Autodesk Inventor part; units mm, degrees
ref_plane "YZ Plane" through (0, 0, 0) normal (1, 0, 0) x (0, 1, 0)
ref_plane "XZ Plane" through (0, 0, 0) normal (0, 1, 0) x (-1, 0, 0)
ref_plane "XY Plane" through (0, 0, 0) normal (0, 0, 1) x (1, 0, 0)
sketch "Эскиз1" plane through (0, 0, 0) normal (0, 0, 1) x (1, 0, 0)
  line L0 (40, 0) -> (0, 0)
  line L1 (40, 0) -> (40, -6)
  line L2 (0, -6) -> (40, -6)
  line L3 (0, 0) -> (0, -6)
  line L4 (0, 0) -> (0, 20)
  line L5 (0, 20) -> (18.33, 29.326)
  line L6 (40, 0) -> (40, 29.326)
  line L7 (40, 29.326) -> (18.33, 29.326)
  dimension "d0" = 20
extrude "Выдавливание1" add sketch "Эскиз1" along normal blind 6
sketch "Эскиз2" plane through (0, 0, 6) normal (0, 0, 1) x (1, 0, 0)
  line L0 (0, 20) -> (0, -6)
  line L1 (40, 29.326) -> (18.33, 29.326)
  line L2 (18.33, 29.326) -> (0, 20)
  line L3 (18.33, 29.326) -> (0, 20)
  line L4 (0, 8.2778) -> (18.33, 29.326)
  point P0 (0, 0)
extrude "Выдавливание2" cut sketch "Эскиз2" against normal blind 6
sketch "Эскиз3" plane through (0, 0, 6) normal (0, 0, 1) x (1, 0, 0)
  line L0 (0, 8.2778) -> (0, -6)
  line L1 (0, 8.2778) -> (34.2751, 29.326)
  line L2 (40, 29.326) -> (18.33, 29.326)
  line L3 (0, 8.2778) -> (18.33, 29.326)
  line L4 (18.33, 29.326) -> (34.2751, 29.326)
  point P0 (0, 0)
extrude "Выдавливание3" cut sketch "Эскиз3" against normal blind 6
sketch "Эскиз4" plane through (0, 0, 0) normal (0, 0, -1) x (-1, 0, 0)
  point P0 (0, 0)
sketch "Эскиз5" plane through (0, 0, 0) normal (0, 0, -1) x (-1, 0, 0)
  line L0 (4.9019, -6) -> (-15.0981, -6)
  line L1 (0, -6) -> (-40, -6)
  point P0 (0, 0)
properties part number "Лепесток"
Design review of the part built by this model. Coordinates are the model's own, in mm. Give positions to 0.01 mm unless a question says otherwise; leave off trailing zeros. Order: outer loops, then holes, each group sorted by start corner. A loop starts at its lowest first (then second) coordinate and runs counter-clockwise, first axis right, second up. Notation, with made-up numbers: (65, 28) - (88, 28) arc R23 cw to (88, 52) - close; hole circle Ø5 at (-24.5, 76.25). An arc over 180 degrees is marked (long way). Use CSV: the item, a comma, the result in double quotes. Start each with the question number.
Q1. Take a section at C-C (x = 24.5). State the section outline as (y, z) points.
Q2. For P1, Ø1.5, axis at x = 20.5, y = 9, coming from the -Z side, flat-tipped, find the tip position at first contact; note if it passes through.
Q3. Take a section at A-A (z = 0.45). State the section outline as (x, y) points.
Q4. Take a section at B-B (y = 23). State the section outline as (x, z) points.
Q5. For line 1 (X direction, y = 8.5, z = 0.45); line 2 (X direction, y = 25.5, z = 4.5); line 3 (Y direction, x = 7.5, z = 4.65), list the stretches that pass through material, from the lowest coordinate up.
Calculated:
1,outline,"(-6, 0) - (23.32, 0) - (23.32, 6) - (-6, 6) - close"
2,P1,"stops at z = 0"
3,outline,"(0, -6) - (40, -6) - (40, 29.33) - (34.28, 29.33) - (0, 8.28) - close"
4,outline,"(23.97, 0) - (40, 0) - (40, 6) - (23.97, 6) - close"
5,line 1,"x = 0.36 to 40"
5,line 2,"x = 28.04 to 40"
5,line 3,"y = -6 to 12.88"
